Geometry: final body of the model. Coordinates: model frame, mm. A direction names the side the tool comes from. Give positions to 0.01 mm unless a question says otherwise; leave off trailing zeros. Write each loop counter-clockwise with the first axis right and the second up, starting at its lowest first coordinate (ties: lowest second). Pieces come first, ordered by that corner, then holes.
```python
from build123d import *

# Parameters (mm, degrees)
F0_R     = 12.5
F0_R_2   = 40
F1_DEPTH = 25


with BuildPart() as f1:
    # F0 (on Front) → F1 (new body)
    with BuildSketch(Plane.XZ):
        with BuildLine():
            ThreePointArc((0, 75), (53.033009, 53.033009), (75, 0))
            ThreePointArc((75, 0), (53.033009, -53.033009), (0, -75))
            Line((0, -75), (200, -75))
            Line((200, -75), (200, -25))
            Line((200, -25), (130, -25))
            Line((130, -25), (130, 25))
            Line((130, 25), (200, 25))
            Line((200, 25), (200, 75))
            Line((200, 75), (0, 75))
        make_face()
        with Locations((165, -50)):
            Circle(F0_R, mode=Mode.SUBTRACT)
        with Locations((165, 50)):
            Circle(F0_R, mode=Mode.SUBTRACT)
        with BuildLine():
            ThreePointArc((0, -75), (53.033009, -53.033009), (75, 0))
            ThreePointArc((75, 0), (53.033009, 53.033009), (0, 75))
            ThreePointArc((0, 75), (-75, 0), (0, -75))
        make_face()
        Circle(F0_R_2, mode=Mode.SUBTRACT)
    extrude(amount=F1_DEPTH)


solid = f1.part
```
Item 1: Section C-C, the plane y = -9.5. Return the cut outline in (x, z), plus the area to 3 significant figures.
Found:
outline: (0, -75) - (200, -75) - (200, -25) - (130, -25) - (130, 25) - (200, 25) - (200, 75) - (0, 75) arc R75 ccw to start; hole circle Ø80 at (0, 0); hole circle Ø25 at (165, -50); hole circle Ø25 at (165, 50)
area: 29,300 mm2
Item 2: Pin query (flat end, axial travel): pin 1 Ø6 at (y, z) = (-17.5, -37) entering from -X; pin 2 Ø2 at (y, z) = (-11.5, 56) entering from -X; pin 3 Ø2 at (y, z) = (-3.5, -33.5) entering from -X. Return the tip coordinate at first contact, or that it passes through.
Found:
pin 1: stops at x = -66.85
pin 2: stops at x = -50.99
pin 3: stops at x = -67.59
Item 3: Line query: L1, parallel to Z at x = 165, y = -17.75; L2, parallel to X at y = -19.5, z = 13.5 (3 decimals); L3, parallel to Z at x = -19, y = -14.25. Output: solid intervals per line, ascending.
Found:
L1: z = -75 to -62.5, -37.5 to -25, 25 to 37.5, 62.5 to 75
L2: x = -73.775 to -37.653, 37.653 to 130
L3: z = -72.55 to -35.2, 35.2 to 72.55
Item 4: Pull-direction query (Z, two-part tool) for faces 1 (the face through (99, -12, -75)), 2 (the face through (165, -12, -25)), 3 (the face through (200, -12, -50)); classes: +Z half, -Z half, draft (parallel to the pull), parting line (faces both ways), or undercut.
Found:
face 1: -Z half
face 2: undercut
face 3: draft
Item 5: Section B-B, the plane z = -21. Return the cut outline in (x, y).
Found:
outline: (-72, -25) - (-34.04, -25) - (-34.04, 0) - (-72, 0) - close; (34.04, -25) - (130, -25) - (130, 0) - (34.04, 0) - close
Item 6: Reachability of faces 4 (the face through (101, -12, 75)), 5 (the face through (130, -12, 0)) from +Z, -Z, +X, -X, +Y, -Y: full face, straight path, thin tool, end or side. Return the list, or none.
Found:
face 4: +Z, +X, -X, +Y, -Y
face 5: +X, +Y, -Y
Item 7: Section A-A, the plane x = -32. Return the cut outline in (y, z).
Found:
outline: (-25, -67.83) - (0, -67.83) - (0, -24) - (-25, -24) - close; (-25, 24) - (0, 24) - (0, 67.83) - (-25, 67.83) - close
Item 8: Section D-D, the plane x = 165. Return the cut outline in (y, z), plus the area to 3 significant figures.
Found:
outline: (-25, -75) - (0, -75) - (0, -62.5) - (-25, -62.5) - close; (-25, -37.5) - (0, -37.5) - (0, -25) - (-25, -25) - close; (-25, 25) - (0, 25) - (0, 37.5) - (-25, 37.5) - close; (-25, 62.5) - (0, 62.5) - (0, 75) - (-25, 75) - close
area: 1,250 mm2
